Work out the finished part from the listing and answer in its coordinate system (mm). Face numbers are marked on the shaded views. A direction names the side the tool comes from. Coordinates: 2 decimals unless noted, no trailing zeros. Write each loop counter-clockwise with the first axis right and the second up, starting at its lowest first coordinate (ties: lowest second). Pieces come first, ordered by that corner, then holes. Notation, with made-up numbers: (28.5, 27.5) - (86.5, 27.5) arc R15 cw to (86.5, 35.5) - close; hole circle Ø10 at (5.5, 16.25). An arc over 180 degrees is marked (long way). Use one line per item in the form item = value. Start each with the question number.
Item 1: A cutting plane is placed at A-A (z = 66). Write down the section's boundary in (x, y), then the cut area to 3 significant figures.
Item 2: A cutting plane is placed at B-B (x = -4). Write down the section's boundary in (y, z), then the cut area to 3 significant figures.
Item 3: Consider probe 1 along Z at (x, y) = (-26, 1.25); probe 2 along X at (y, z) = (2.7, 66); probe 3 along X at (y, z) = (2.6, -9). Determine where each line is inside the solid, lowest interval first.
Item 4: Given pin 1 (1 mm diameter, centred on x = -9.5, z = -1.5, fed in from +Y); pin 2 (2 mm diameter, centred on y = 2.5, z = -16, fed in from +X); pin 3 (1.7 mm diameter, centred on x = -4, z = 66, fed in from -Y); pin 4 (0.5 mm diameter, centred on y = 2.5, z = -14.5, fed in from -X), each flat-ended and moving along its own axis, determine where each tip first touches the part or whether it passes through.
Item 5: A cutting plane is placed at D-D (z = -14). Write down the section's boundary in (x, y), then the cut area to 3 significant figures.
Item 6: For the marked faces 1, 2 and 3, determine the directions among +Z, -Z, +X, -X, +Y, -Y from which every point of the face is accessible in a straight line to the end or side of a thin tool.
Item 7: A cutting plane is placed at C-C (x = -18.5). Write down the section's boundary in (y, z), then the cut area to 3 significant figures.
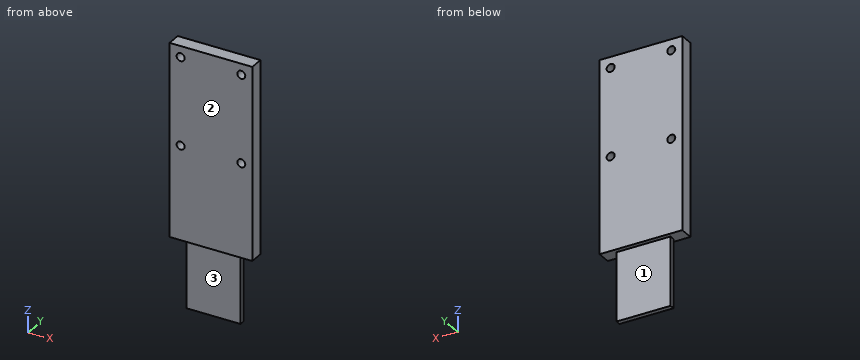
from build123d import *

# Parameters (mm, degrees)
SKETCH_1_W          = 30
SKETCH_1_H          = 5
EXTRUDE_1_DEPTH     = 70
SKETCH_2_R          = 1.45
CUT_EXTRUDE_1_DEPTH = 60
SKETCH_4_W          = 19.6
SKETCH_4_H          = 1.8
EXTRUDE_2_DEPTH     = 25


with BuildPart() as part:
    # 草图1 → 凸台-拉伸1 (new body)
    with BuildSketch(Plane.XY):
        with Locations((-15, 2.5)):
            Rectangle(SKETCH_1_W, SKETCH_1_H)
    extrude(amount=EXTRUDE_1_DEPTH)

    # 草图2 → 切除-拉伸1 (cut)
    with BuildSketch(Plane(origin=(0, 5, 0), x_dir=(1, 0, 0), z_dir=(0, 1, 0))):
        with Locations(Location((-26, -66, 0), (0, 0, 180))):
            Circle(SKETCH_2_R)
        with Locations(Location((-26, -34.1, 0), (0, 0, 180))):
            Circle(SKETCH_2_R)
        with Locations(Location((-4, -66, 0), (0, 0, 270))):
            Circle(SKETCH_2_R)
        with Locations(Location((-4, -34.1, 0), (0, 0, 270))):
            Circle(SKETCH_2_R)
    extrude(amount=-CUT_EXTRUDE_1_DEPTH, mode=Mode.SUBTRACT)

    # 草图4 → 凸台-拉伸2 (add)
    with BuildSketch(Plane(origin=(0, 0, 0), x_dir=(-1, 0, 0), z_dir=(0, 0, -1))):
        with Locations((15, 2.5)):
            Rectangle(SKETCH_4_W, SKETCH_4_H)
    extrude(amount=EXTRUDE_2_DEPTH)


solid = part.part
Answer:
q1.outline = (-30, 0) - (-27.45, 0) - (-27.45, 5) - (-30, 5) - close; (-24.55, 0) - (-5.45, 0) - (-5.45, 5) - (-24.55, 5) - close; (-2.55, 0) - (0, 0) - (0, 5) - (-2.55, 5) - close
q1.area = 121 mm²
q2.outline = (0, 0) - (5, 0) - (5, 32.65) - (0, 32.65) - close; (0, 35.55) - (5, 35.55) - (5, 64.55) - (0, 64.55) - close; (0, 67.45) - (5, 67.45) - (5, 70) - (0, 70) - close
q2.area = 321 mm²
q3.probe_1 = 0 to 32.65, 35.55 to 64.55, 67.45 to 70
q3.probe_2 = -30 to -27.45, -24.55 to -5.45, -2.55 to 0
q3.probe_3 = -24.8 to -5.2
q4.pin_1 = 3.4
q4.pin_2 = -5.2
q4.pin_3 = through
q4.pin_4 = -24.8
q5.outline = (-24.8, 1.6) - (-5.2, 1.6) - (-5.2, 3.4) - (-24.8, 3.4) - close
q5.area = 35.3 mm²
q6.face_1 = -Z, +X, -X, +Y
q6.face_2 = +Z, -Z, +X, -X, -Y
q6.face_3 = -Z, +X, -X, -Y
q7.outline = (0, 0) - (1.6, 0) - (1.6, -25) - (3.4, -25) - (3.4, 0) - (5, 0) - (5, 70) - (0, 70) - close
q7.area = 395 mm²
